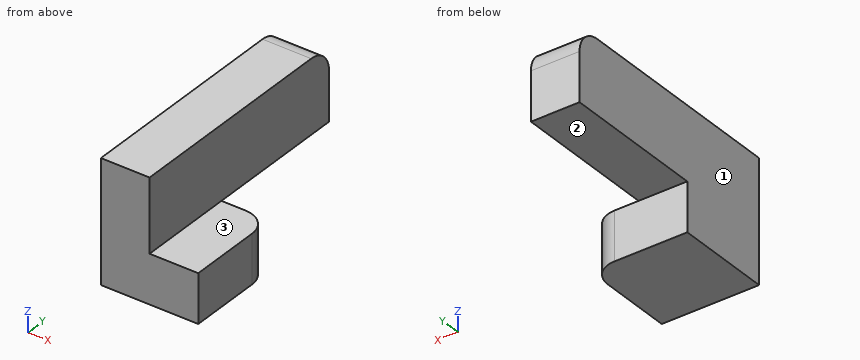
from build123d import *

# Parameters (mm, degrees)
SKETCH1_W           = 20
SKETCH1_H           = 100
BOSS_EXTRUDE1_DEPTH = 30
SKETCH2_W           = 40
SKETCH2_H           = 40
BOSS_EXTRUDE2_DEPTH = 20
FILLET1_R           = 10


with BuildPart() as part:
    # Sketch1 → Boss-Extrude1 (new body)
    with BuildSketch(Plane.XY):
        with Locations((-20, -50)):
            Rectangle(SKETCH1_W, SKETCH1_H)
    extrude(amount=BOSS_EXTRUDE1_DEPTH)

    # Sketch2 → Boss-Extrude2 (add)
    with BuildSketch(Plane.XY):
        with Locations((-10, -80)):
            Rectangle(SKETCH2_W, SKETCH2_H)
    extrude(amount=-BOSS_EXTRUDE2_DEPTH)

    # Fillet1
    fillet1_edges = [part.edges().sort_by_distance(p)[0] for p in [
        (10, -60, -10),
        (-20, 0, 30),
    ]]
    fillet(fillet1_edges, radius=FILLET1_R)


solid = part.part
Design review of the part built by this model. Coordinates are the model's own, in mm. Face numbers are marked on the shaded views. A direction names the side the tool comes from. Coordinates: 2 decimals unless noted, no trailing zeros. Write each loop counter-clockwise with the first axis right and the second up, starting at its lowest first coordinate (ties: lowest second). Pieces come first, ordered by that corner, then holes. Notation, with made-up numbers: (-17.5, -19) -> (29.5, -19) arc R18 cw to (29.5, 12) -> close; hole circle Ø3 at (35.25, -20.5). An arc over 180 degrees is marked (long way). Write each question's results on one line, items separated by ' | '. Start each with the question number.
(1) Clearance check with flat-ended pins moving along their axes: P1, Ø6, axis at x = 4, y = -90, coming from the +Z side; P2, Ø8, axis at y = -34, z = 19.5, coming from the +X side; P3, Ø1, axis at x = -13.5, z = 22.5, coming from the +Y side; P4, Ø16, axis at x = -15, z = -6, coming from the +Y side. State where each tip first meets the part, or that it passes through.
(2) Take a section at A-A on x = -23. Write out the cut boundary in (y, z).
(3) Take a section at C-C on z = -2.5. Write out the cut boundary in (x, y).
(4) Tool access review of the marked faces 1, 2 and 3: name each direction out of +Z, -Z, +X, -X, +Y, -Y from which nothing blocks a thin tool from reaching the whole face with its end or side.
(5) Take a section at D-D on y = -92. Write out the cut boundary in (x, z).
(6) Take a section at B-B on y = -14. Write out the cut boundary in (x, z).
(7) For line 1 along Z through (x, y) = (-15.5, -45.5); line 2 along Y through (x, z) = (-18, -17.5); line 3 along X through (y, z) = (-47, 22.5), list the stretches that pass through material, from the lowest coordinate up. Write a range as from..to.
Results found:
1) P1: stops at z = 0 | P2: stops at x = -10 | P3: stops at y = -0.2 | P4: stops at y = 0
2) outline: (-100, -20) -> (-60, -20) -> (-60, 0) -> (0, 0) -> (0, 20) arc R10 ccw to (-10, 30) -> (-100, 30) -> close
3) outline: (-30, -100) -> (10, -100) -> (10, -70) arc R10 ccw to (0, -60) -> (-30, -60) -> close
4) face 1: +Z, -Z, -X, +Y, -Y | face 2: -Z, +X, -X, +Y | face 3: +Z, +X, +Y, -Y
5) outline: (-30, -20) -> (10, -20) -> (10, 0) -> (-10, 0) -> (-10, 30) -> (-30, 30) -> close
6) outline: (-30, 0) -> (-10, 0) -> (-10, 30) -> (-30, 30) -> close
7) line 1: z = 0..30 | line 2: y = -100..-60 | line 3: x = -30..-10
